The model under review builds one solid part; all positions refer to its coordinate system, in mm. A direction names the side the tool comes from. Coordinates: 2 decimals unless noted, no trailing zeros. Order: outer loops, then holes, each group sorted by start corner. A loop starts at its lowest first (then second) coordinate and runs counter-clockwise, first axis right, second up.
```python
from build123d import *

# Parameters (mm, degrees)
F0_R            = 2.15265
F1_DEPTH        = 12.7
F2_R            = 2.15265
F3_REACH        = 42.6021136501
F5_R            = 3.96875
F6_DEPTH        = 6.35
F8_DEPTH        = 12.7
F8_COPIES_COUNT = 3
F8_COPIES_ANGLE = 180


# Not quite as in the source:
# - a pattern or mirror of a feature is missing from the dataset's text; its kind, count and spacing are read off the source's solid


with BuildPart() as f1:
    # F0 (on Top) → F1 (new body)
    with BuildSketch(Plane.XY):
        with BuildLine():
            Line((3.96875, 14.2875), (0, 14.2875))
            Line((0, 14.2875), (-3.96875, 14.2875))
            Line((-3.96875, 14.2875), (-3.96875, 21.8677764859))
            ThreePointArc((-3.96875, 21.8677764859), (0, -22.225), (3.96875, 21.8677764859))
            Line((3.96875, 21.8677764859), (3.96875, 14.2875))
        make_face()
        with Locations((-11.7865861589, -11.7865861589)):
            Circle(F0_R, mode=Mode.SUBTRACT)
        with Locations((11.7865861589, -11.7865861589)):
            Circle(F0_R, mode=Mode.SUBTRACT)
        with Locations((-11.7865861589, 11.7865861589)):
            Circle(F0_R, mode=Mode.SUBTRACT)
        with BuildLine():
            ThreePointArc((0, 11.1125), (7.8577241059, 7.8577241059), (11.1125, 0))
            ThreePointArc((11.1125, 0), (-7.8577241059, -7.8577241059), (0, 11.1125))
        make_face(mode=Mode.SUBTRACT)
        with Locations((11.7865861589, 11.7865861589)):
            Circle(F0_R, mode=Mode.SUBTRACT)
    extrude(amount=F1_DEPTH)

    f3_end = f1.faces().sort_by_distance((0, -11.1125, 6.35))[0]
    # F2 (on face) → F3 (cut, up to a face of the model that its end follows)
    with BuildSketch(Plane(origin=(0, 14.2875, 0), x_dir=(-1, 0, 0), z_dir=(0, 1, 0))):
        with Locations((0, 6.35)):
            Circle(F2_R)
    f3_long = extrude(amount=-F3_REACH, mode=Mode.PRIVATE)
    add(split(f3_long, bisect_by=f3_end, keep=Keep.ALL, mode=Mode.PRIVATE).solids().sort_by_distance((0, 14.2875, 6.35))[0], mode=Mode.SUBTRACT)

    # F5 (on face) → F6 (cut, through all)
    with BuildSketch(Plane(origin=(0, 0, 0), x_dir=(1, 0, 0), z_dir=(0, 0, -1))):
        with Locations((11.7865861589, -11.7865861589)):
            Circle(F5_R)
        with Locations((-11.7865861589, 11.7865861589)):
            Circle(F5_R)
    extrude(amount=-F6_DEPTH, mode=Mode.SUBTRACT)

    # F7 (on face) → F8 (cut, through all)
    with BuildSketch(Plane(origin=(0, 0, 0), x_dir=(1, 0, 0), z_dir=(0, 0, -1))):
        with BuildLine():
            ThreePointArc((-17.3148424047, -11.229543123), (-15.8788163052, -8.0281867), (-12.8109235396, -6.3255746232))
            ThreePointArc((-12.8109235396, -6.3255746232), (-14.2875, 0), (-12.8109235396, 6.3255746232))
            ThreePointArc((-12.8109235396, 6.3255746232), (-15.8788163052, 8.0281867), (-17.3148424047, 11.229543123))
            ThreePointArc((-17.3148424047, 11.229543123), (-20.6375, 0), (-17.3148424047, -11.229543123))
        make_face()
    f8 = extrude(amount=-F8_DEPTH, mode=Mode.SUBTRACT)

    # F8_copies: F8 ×3 about axis
    f8_copies_axis = Axis((0, 0, 0), (0, 0, 1))
    for i in range(1, F8_COPIES_COUNT):
        add(f8.rotate(f8_copies_axis, i * F8_COPIES_ANGLE / (F8_COPIES_COUNT - 1)), mode=Mode.SUBTRACT)


solid = f1.part
```
(1) For pin 1 Ø5 at (x, y) = (11.79, 11.79) entering from -Z; pin 2 Ø1.5 at (x, z) = (-7.5, 3.5) entering from -Y; pin 3 Ø2.5 at (x, z) = (1.5, 5.5) entering from +Y, all flat-tipped, find the tip position at first contact; note any pin that passes through.
A:
pin 1: stops at z = 6.35
pin 2: stops at y = -21.18
pin 3: stops at y = 14.29
(2) Machinability: for faces 4 (the face through (-3.969, 18, 6)), 5 (the face through (10.2, -10.33, 6.26)), 6 (the face through (0.47, 12.62, 4.25)), 7 (the face through (-10, -10, 6.35)), which of the approach directions +Z, -Z, +X, -X, +Y, -Y give a long, thin tool a straight path to every point of the face, cutting with its end or side? Answer none if there is none.
A:
face 4: +Z, -Z, +Y
face 5: +Z, -Z
face 6: +Y
face 7: -Z
(3) We need section A-A, the plane y = 5.5. Write out the cut boundary in (x, z).
A:
outline: (-21.53, 0) - (-19.89, 0) - (-19.89, 12.7) - (-21.53, 12.7) - close; (-13.19, 0) - (-9.66, 0) - (-9.66, 12.7) - (-13.19, 12.7) - close; (9.66, 0) - (13.19, 0) - (13.19, 12.7) - (9.66, 12.7) - close; (19.89, 0) - (21.53, 0) - (21.53, 12.7) - (19.89, 12.7) - close
(4) Wall thickness on probe 1 along X at (y, z) = (10, 9.5); probe 2 along Y at (x, z) = (3, 1); probe 3 along Y at (x, z) = (-11.5, 10.5): over which ranges is each line inside the solid? List them lowest first.
A:
probe 1: x = -19.85 to -18.05, -17.05 to -12.99, -10.59 to -4.85, 4.85 to 10.59, 12.99 to 17.05, 18.05 to 19.85
probe 2: y = -22.02 to -20.42, -13.97 to -10.7, 10.7 to 14.29
probe 3: y = -19.02 to -13.92, -9.65 to 9.65, 13.92 to 19.02
(5) We need section B-B, the plane x = 1.5. Write out the cut boundary in (y, z).
A:
outline: (-22.17, 0) - (-20.58, 0) - (-20.58, 12.7) - (-22.17, 12.7) - close; (-14.21, 0) - (-11.01, 0) - (-11.01, 12.7) - (-14.21, 12.7) - close; (11.01, 0) - (14.29, 0) - (14.29, 4.81) - (11.01, 4.81) - close; (11.01, 7.89) - (14.29, 7.89) - (14.29, 12.7) - (11.01, 12.7) - close
(6) We need section C-C, the plane y = -15. Write out the cut boundary in (x, z).
A:
outline: (-16.4, 0) - (-14.12, 0) - (-14.12, 6.35) - (-9.46, 6.35) - (-9.46, 0) - (-7.25, 0) - (-7.25, 12.7) - (-16.4, 12.7) - close; (7.25, 0) - (16.4, 0) - (16.4, 12.7) - (7.25, 12.7) - close
(7) Draft analysis for pull direction Y (two halves, no side actions). For faces 1 (the face through (-0.1, 11.4, 0)), 2 (the face through (-2, 14.288, 8)), 3 (the face through (-8, -12.98, 3.13)), state which applies: released by +Y, released by -Y, zero draft, split by the parting line, or undercut.
A:
face 1: zero draft
face 2: released by +Y
face 3: undercut
